```python
from build123d import *

# Parameters (mm, degrees)
EXTRUDE_THIN1_DEPTH            = 80
SKETCH4_W                      = 80
SKETCH4_H                      = 80
BOSS_EXTRUDE1_DEPTH            = 80
SKETCH5_R                      = 35
CUT_EXTRUDE1_DEPTH             = 1
CUT_EXTRUDE1_DEPTH_BACK        = 74
CBORE_FOR_M4_SHCS1_D           = 4.5
CBORE_FOR_M4_SHCS1_DEPTH       = 6
CBORE_FOR_M4_SHCS1_CBORE_D     = 8
CBORE_FOR_M4_SHCS1_CBORE_DEPTH = 4


with BuildPart() as part:
    # Sketch1 → Extrude-Thin1 (new body)
    with BuildSketch(Plane(origin=(0, 0, 0), x_dir=(0, 0, -1), z_dir=(1, 0, 0))):
        Polygon((0, -40), (0, 0), (-40, 0), (-40, 6), (6, 6), (6, -40), align=None)
    extrude(amount=EXTRUDE_THIN1_DEPTH)

    # Sketch4 → Boss-Extrude1 (add)
    with BuildSketch(Plane(origin=(0, 6, 0), x_dir=(1, 0, 0), z_dir=(0, 1, 0))):
        with Locations((40, 40)):
            Rectangle(SKETCH4_W, SKETCH4_H)
    extrude(amount=-BOSS_EXTRUDE1_DEPTH)

    # Sketch5 → Cut-Extrude1 (cut, two sides)
    with BuildSketch(Plane(origin=(0, 6, 0), x_dir=(1, 0, 0), z_dir=(0, 1, 0))) as cut_extrude1_sk:
        with Locations((40, 40)):
            Circle(SKETCH5_R)
    extrude(amount=CUT_EXTRUDE1_DEPTH, mode=Mode.SUBTRACT)
    extrude(cut_extrude1_sk.sketch, amount=-CUT_EXTRUDE1_DEPTH_BACK, mode=Mode.SUBTRACT)

    # CBORE for M4 SHCS1
    with Locations(Plane(origin=(0, 6, 0), x_dir=(1, 0, 0), z_dir=(0, 1, 0))):
        with Locations((60, -20), (20, -20)):
            CounterBoreHole(CBORE_FOR_M4_SHCS1_D / 2, CBORE_FOR_M4_SHCS1_CBORE_D / 2, CBORE_FOR_M4_SHCS1_CBORE_DEPTH, depth=CBORE_FOR_M4_SHCS1_DEPTH)


solid = part.part
```
Source: CAD feature listing. Evaluate the final solid. Frame: model axes, mm. A direction names the side the tool comes from. Coordinates: 2 decimals unless noted, no trailing zeros. Loops run counter-clockwise (first coordinate to the right, second up) from the corner with the lowest first, then second, coordinate; pieces in that order, holes last. Notation, with made-up numbers: M -21.5,60.5 L -15.5,60.5 A27 ccw -15.5,98.5 Z; hole C 27,9 d5. An arc over 180 degrees is marked long. Use a Markdown table: item, result. Add a question column.
Q1. Section query C-C, the plane z = -40. Return loops of the section in (x, y), and give its area (3 significant figures).
Q2. Section query A-A, the plane z = 20. Return loops of the section in (x, y).
Q3. Access query for faces 1 (the flat face through (31, 6, -6)), 2 (the flat face through (62, 2, 22)), 3 (the flat face through (39, -38, 0)). Directions: +Z, -Z, +X, -X, +Y, -Y. A direction counts if a zero-diameter tool reaches every point of the face in a straight line with its end or side. Return the directions, or none.
Q4. Section query D-D, the plane x = 60. Return loops of the section in (y, z).
Q5. First-contact query: pin 1 (6.5 mm diameter, centred on x = 20, z = 20, fed in from -Y); pin 2 (5 mm diameter, centred on x = 60, z = 20, fed in from +Y); pin 3 (3 mm diameter, centred on x = 17, z = -62.5, fed in from +Y). Flat tips, straight axial feed; report the tip coordinate or a pass-through.
Q6. Draft query along Z for faces 4 (the cylindrical face through (61.786, 0.986, 21.369)), 5 (the flat face through (39, 3, 40)), 6 (the flat face through (39, 0, 20)). Return one class per face: pulls with the +Z half, pulls with the -Z half, needs draft (parallel to the pull), parting line crosses it, or undercut.
Q7. Material intervals for L1, parallel to X at y = 4.75, z = 20; L2, parallel to X at y = 0.45, z = 20; L3, parallel to Z at x = 20, y = 4.9, sorted ascending.
Q8. Section query B-B, the plane y = -47. Return loops of the section in (x, z).
Result:
| question | item | result |
|---|---|---|
| 1 | outline | M 0,-74 L 80,-74 L 80,6 L 75,6 L 75,-68 L 5,-68 L 5,6 L 0,6 Z |
| 1 | area | 1,220 mm2 |
| 2 | outline | M 0,0 L 17.75,0 L 17.75,2 L 16,2 L 16,6 L 0,6 Z; M 22.25,0 L 57.75,0 L 57.75,2 L 56,2 L 56,6 L 24,6 L 24,2 L 22.25,2 Z; M 62.25,0 L 80,0 L 80,6 L 64,6 L 64,2 L 62.25,2 Z |
| 3 | face 1 | +Z, -Z, +X, -X, +Y |
| 3 | face 2 | +Y |
| 3 | face 3 | +Z, +X, -X, -Y |
| 4 | outline | M -74,-80 L 6,-80 L 6,-68.72 L -68,-68.72 L -68,-11.28 L 6,-11.28 L 6,16 L 2,16 L 2,17.75 L 0,17.75 L 0,0 L -74,0 Z; M 0,22.25 L 2,22.25 L 2,24 L 6,24 L 6,40 L 0,40 Z |
| 5 | pin 1 | stops at y = 0 |
| 5 | pin 2 | stops at y = 2 |
| 5 | pin 3 | stops at y = -68 |
| 6 | face 4 | undercut |
| 6 | face 5 | pulls with the +Z half |
| 6 | face 6 | needs draft |
| 7 | L1 | x = 0 to 16, 24 to 56, 64 to 80 |
| 7 | L2 | x = 0 to 17.75, 22.25 to 57.75, 62.25 to 80 |
| 7 | L3 | z = -80 to -68.72, -11.28 to 16, 24 to 40 |
| 8 | outline | M 0,-80 L 80,-80 L 80,0 L 0,0 Z; hole C 40,-40 d70 |
